Part model, mm, in its own coordinate system. Face numbers are marked on the shaded views. A direction names the side the tool comes from. Give positions to 0.01 mm unless a question says otherwise; leave off trailing zeros. Order: outer loops, then holes, each group sorted by start corner. A loop starts at its lowest first (then second) coordinate and runs counter-clockwise, first axis right, second up. Notation, with made-up numbers: (44.5, -28.75) - (89.5, -28.75) arc R18 cw to (89.5, -0.75) - close; hole circle Ø9 at (6.5, 0.5). An arc over 180 degrees is marked (long way). Use one line per item in the form item = value. Start each with the question number.
1. Tool access for the marked faces 1, 2 and 3: list every direction of +Z, -Z, +X, -X, +Y, -Y with a clear straight run to the whole face (end or side of a thin tool).
2. Band-saw the part on D-D, the plane x = 0. List the corners of the cut face in (y, z), plus the area to 3 significant figures.
3. Pull direction Z, two halves, no side cores. Call the marked faces 4, 5 and 6: +Z half, -Z half, draft (parallel to the pull), parting line (faces both ways), or undercut.
4. Pin check, flat tips, straight feed: P1, Ø4.5, axis at x = 0, z = -37.5, coming from the -Y side; P2, Ø2, axis at y = 2.5, z = 6.5, coming from the +X side; P3, Ø1.5, axis at x = -28.5, y = 1, coming from the +Z side. Stop position of each tip, or through.
5. Band-saw the part on C-C, the plane x = 7.5. List the corners of the cut face in (y, z).
6. Band-saw the part on B-B, the plane y = 1.3. List the corners of the cut face in (x, z), plus the area to 3 significant figures.
7. Drill centre lines: line 1 (Z direction, x = 1, y = 5.1); line 2 (X direction, y = 3.3, z = 14.5); line 3 (X direction, y = 5.25, z = 2.5). Where is each one in solid material? Low to high.
8. Band-saw the part on A-A, the plane z = 6. List the corners of the cut face in (x, y), plus the area to 3 significant figures.
from build123d import *

# Parameters (mm, degrees)
SKETCH1_R                = 17.5
BOSS_EXTRUDE1_DEPTH      = 5.5
SKETCH2_R                = 35
SKETCH2_R_2              = 17.5
SKETCH2_R_3              = 2.8
BOSS_EXTRUDE2_DEPTH      = 5.5
BOSS_EXTRUDE3_DEPTH      = 2
BOSS_EXTRUDE3_DEPTH_BACK = 5.5
SKETCH4_R                = 2.9
SKETCH5_R                = 5
BOSS_EXTRUDE4_DEPTH      = 1.5
SKETCH3_R                = 17.5
CUT_EXTRUDE1_DEPTH       = 10
SKETCH12_R               = 72.135852014
CUT_EXTRUDE2_DEPTH       = 22
FILLET1_R                = 10
SKETCH13_R               = 3.4
CUT_EXTRUDE3_DEPTH       = 10
SKETCH14_R               = 19
CUT_EXTRUDE4_DEPTH       = 10


with BuildPart() as part:
    # Sketch1 → Boss-Extrude1 (new body)
    with BuildSketch(Plane(origin=(0, 0, 0), x_dir=(1, 0, 0), z_dir=(0, 1, 0))):
        with Locations(Location((0, 0, 0), (0, 0, 270))):
            Circle(SKETCH1_R)
    extrude(amount=BOSS_EXTRUDE1_DEPTH)

    # Sketch2 → Boss-Extrude2 (add)
    with BuildSketch(Plane(origin=(0, 0, 0), x_dir=(1, 0, 0), z_dir=(0, 1, 0))):
        with Locations(Location((0, 0, 0), (0, 0, 270))):
            Circle(SKETCH2_R)
        Circle(SKETCH2_R_2, mode=Mode.SUBTRACT)
        with Locations(Location((0, 29, 0), (0, 0, 270))):
            Circle(SKETCH2_R_3, mode=Mode.SUBTRACT)
        with Locations(Location((25.11473671, -14.5, 0), (0, 0, 270))):
            Circle(SKETCH2_R_3, mode=Mode.SUBTRACT)
        with Locations(Location((-25.11473671, -14.5, 0), (0, 0, 270))):
            Circle(SKETCH2_R_3, mode=Mode.SUBTRACT)
    extrude(amount=BOSS_EXTRUDE2_DEPTH)

    # Sketch4 → Boss-Extrude3 (add, two sides: drawn at the far end of the back side and taken through both)
    with BuildSketch(Plane.XZ.offset(-BOSS_EXTRUDE3_DEPTH_BACK)):
        with Locations(Location((-25.11473671, 14.5, 0), (0, 0, 270))):
            Circle(SKETCH4_R)
        with Locations(Location((25.11473671, 14.5, 0), (0, 0, 270))):
            Circle(SKETCH4_R)
        with Locations(Location((0, -29, 0), (0, 0, 270))):
            Circle(SKETCH4_R)
    extrude(amount=BOSS_EXTRUDE3_DEPTH + BOSS_EXTRUDE3_DEPTH_BACK)

    # Sketch5 → Boss-Extrude4 (add)
    with BuildSketch(Plane(origin=(0, 5.5, 0), x_dir=(1, 0, 0), z_dir=(0, 1, 0))):
        with Locations((-30.453629482, -17.250404383)):
            Circle(SKETCH5_R)
        with Locations((0.28752632, 34.99881896)):
            Circle(SKETCH5_R)
        with Locations((30.166103162, -17.748414577)):
            Circle(SKETCH5_R)
    extrude(amount=-BOSS_EXTRUDE4_DEPTH)

    # Sketch3 → Cut-Extrude1 (cut)
    with BuildSketch(Plane(origin=(0, 5.5, 0), x_dir=(1, 0, 0), z_dir=(0, 1, 0))):
        with Locations(Location((0, 0, 0), (0, 0, 270))):
            Circle(SKETCH3_R)
    extrude(amount=-CUT_EXTRUDE1_DEPTH, mode=Mode.SUBTRACT)

    # Sketch12 → Cut-Extrude2 (cut)
    with BuildSketch(Plane(origin=(0, 5.5, 0), x_dir=(1, 0, 0), z_dir=(0, 1, 0))):
        Circle(SKETCH12_R)
        Polygon((0, 50), (-43.301270189, -25), (43.301270189, -25), align=None, mode=Mode.SUBTRACT)
    extrude(amount=-CUT_EXTRUDE2_DEPTH, mode=Mode.SUBTRACT)

    # Fillet1
    # the kernel refuses this fillet: 10 mm, written as the material it takes off along each edge
    with BuildSketch(Plane(origin=(-24.494897428, 18.7960859, 25), x_dir=(1, 0, 0), z_dir=(0, -1, 0))) as fillet1_piece_1_section:
        with BuildLine():
            CenterArc((4.494897428, -10), FILLET1_R, 90, 53.130102354)
            ThreePointArc((-3.505102572, -4), (-1.828638885, -1.933326291), (0, 0))
            Line((0, 0), (4.494897428, 0))
        make_face()
    fillet1_piece_1 = extrude(amount=32.0921718, mode=Mode.PRIVATE)
    fillet1_piece_1 = fillet1_piece_1 - Plane(origin=(-30.453629482, 4.75, 17.250404383), x_dir=(1, 0, 0), z_dir=(0, 1, 0)) * Cylinder(5, 83, mode=Mode.PRIVATE)
    add(fillet1_piece_1, mode=Mode.SUBTRACT)
    with BuildSketch(Plane(origin=(-24.494897428, 18.7960859, 25), x_dir=(1, 0, 0), z_dir=(0, -1, 0))) as fillet1_piece_2_section:
        with BuildLine():
            CenterArc((4.494897428, -10), FILLET1_R, 90, 53.130102354)
            ThreePointArc((-3.505102572, -4), (-1.828638885, -1.933326291), (0, 0))
            Line((0, 0), (4.494897428, 0))
        make_face()
    fillet1_piece_2 = extrude(amount=32.0921718, mode=Mode.PRIVATE)
    fillet1_piece_2 = split(fillet1_piece_2, bisect_by=Plane(origin=(-27.761621835, 4, 21.309124186), z_dir=(0, -1, 0)), keep=Keep.TOP, mode=Mode.PRIVATE)
    add(fillet1_piece_2, mode=Mode.SUBTRACT)
    with BuildSketch(Plane(origin=(24.494897428, 18.7960859, 25), x_dir=(-1, 0, 0), z_dir=(0, -1, 0))) as fillet1_piece_3_section:
        with BuildLine():
            CenterArc((4.494897428, 10), FILLET1_R, 216.869897646, 53.130102354)
            ThreePointArc((-3.505102572, 4), (-1.828638885, 1.933326291), (0, 0))
            Line((0, 0), (4.494897428, 0))
        make_face()
    fillet1_piece_3 = extrude(amount=32.0921718, mode=Mode.PRIVATE)
    fillet1_piece_3 = fillet1_piece_3 - Plane(origin=(30.166103162, 4.75, 17.748414577), x_dir=(1, 0, 0), z_dir=(0, 1, 0)) * Cylinder(5, 83, mode=Mode.PRIVATE)
    add(fillet1_piece_3, mode=Mode.SUBTRACT)
    with BuildSketch(Plane(origin=(24.494897428, 18.7960859, 25), x_dir=(-1, 0, 0), z_dir=(0, -1, 0))) as fillet1_piece_4_section:
        with BuildLine():
            CenterArc((4.494897428, 10), FILLET1_R, 216.869897646, 53.130102354)
            ThreePointArc((-3.505102572, 4), (-1.828638885, 1.933326291), (0, 0))
            Line((0, 0), (4.494897428, 0))
        make_face()
    fillet1_piece_4 = extrude(amount=32.0921718, mode=Mode.PRIVATE)
    fillet1_piece_4 = split(fillet1_piece_4, bisect_by=Plane(origin=(27.488157838, 4, 21.643747381), z_dir=(0, -1, 0)), keep=Keep.TOP, mode=Mode.PRIVATE)
    add(fillet1_piece_4, mode=Mode.SUBTRACT)
    with BuildSketch(Plane(origin=(-9.403186381, 18.7960859, -33.713203436), x_dir=(-0.5000000000000003, 0, 0.8660254037844386), z_dir=(0, -1, 0))) as fillet1_piece_5_section:
        with BuildLine():
            CenterArc((4.494897428, -10), FILLET1_R, 90, 53.130102354)
            ThreePointArc((-3.505102572, -4), (-1.828638885, -1.933326291), (0, 0))
            Line((0, 0), (4.494897428, 0))
        make_face()
    fillet1_piece_5 = extrude(amount=32.0921718, mode=Mode.PRIVATE)
    fillet1_piece_5 = fillet1_piece_5 - Plane(origin=(0.28752632, 4.75, -34.99881896), x_dir=(1, 0, 0), z_dir=(0, 1, 0)) * Cylinder(5, 83, mode=Mode.PRIVATE)
    add(fillet1_piece_5, mode=Mode.SUBTRACT)
    with BuildSketch(Plane(origin=(-9.403186381, 18.7960859, -33.713203436), x_dir=(-0.5000000000000003, 0, 0.8660254037844386), z_dir=(0, -1, 0))) as fillet1_piece_6_section:
        with BuildLine():
            CenterArc((4.494897428, -10), FILLET1_R, 90, 53.130102354)
            ThreePointArc((-3.505102572, -4), (-1.828638885, -1.933326291), (0, 0))
            Line((0, 0), (4.494897428, 0))
        make_face()
    fillet1_piece_6 = extrude(amount=32.0921718, mode=Mode.PRIVATE)
    fillet1_piece_6 = split(fillet1_piece_6, bisect_by=Plane(origin=(-4.57343196, 4, -34.696831852), z_dir=(0, -1, 0)), keep=Keep.TOP, mode=Mode.PRIVATE)
    add(fillet1_piece_6, mode=Mode.SUBTRACT)
    with BuildSketch(Plane(origin=(-33.898083809, 18.7960859, 8.713203436), x_dir=(0.32181469455231854, 0, 0.9468026734067654), z_dir=(0, -1, 0))) as fillet1_piece_7_section:
        with BuildLine():
            CenterArc((4.558658023, -9.971095222), FILLET1_R, 85.642603122, 53.130102354)
            Line((-2.962352352, -3.380617019), (0, 0))
            ThreePointArc((0, 0), (2.65921718, 0.101166725), (5.31843436, 0))
        make_face()
    fillet1_piece_7 = extrude(amount=32.0921718, mode=Mode.PRIVATE)
    fillet1_piece_7 = fillet1_piece_7 - Plane(origin=(-30.453629482, 4.75, 17.250404383), x_dir=(1, 0, 0), z_dir=(0, 1, 0)) * Cylinder(5, 86, mode=Mode.PRIVATE)
    add(fillet1_piece_7, mode=Mode.SUBTRACT)
    with BuildSketch(Plane(origin=(-33.898083809, 18.7960859, 8.713203436), x_dir=(0.32181469455231854, 0, 0.9468026734067654), z_dir=(0, -1, 0))) as fillet1_piece_8_section:
        with BuildLine():
            CenterArc((4.558658023, -9.971095222), FILLET1_R, 85.642603122, 53.130102354)
            Line((-2.962352352, -3.380617019), (0, 0))
            ThreePointArc((0, 0), (2.65921718, 0.101166725), (5.31843436, 0))
        make_face()
    fillet1_piece_8 = extrude(amount=32.0921718, mode=Mode.PRIVATE)
    fillet1_piece_8 = split(fillet1_piece_8, bisect_by=Plane(origin=(-32.488113984, 4, 12.9835693), z_dir=(0, -1, 0)), keep=Keep.TOP, mode=Mode.PRIVATE)
    add(fillet1_piece_8, mode=Mode.SUBTRACT)
    with BuildSketch(Plane(origin=(33.898083809, 18.7960859, 8.713203436), x_dir=(-0.5000000000000012, 0, -0.8660254037844382), z_dir=(0, -1, 0))) as fillet1_piece_9_section:
        with BuildLine():
            CenterArc((4.494897428, -10), FILLET1_R, 90, 53.130102354)
            ThreePointArc((-3.505102572, -4), (-1.828638885, -1.933326291), (0, 0))
            Line((0, 0), (4.494897428, 0))
        make_face()
    fillet1_piece_9 = extrude(amount=32.0921718, mode=Mode.PRIVATE)
    fillet1_piece_9 = fillet1_piece_9 - Plane(origin=(30.166103162, 4.75, 17.748414577), x_dir=(1, 0, 0), z_dir=(0, 1, 0)) * Cylinder(5, 83, mode=Mode.PRIVATE)
    add(fillet1_piece_9, mode=Mode.SUBTRACT)
    with BuildSketch(Plane(origin=(33.898083809, 18.7960859, 8.713203436), x_dir=(-0.5000000000000012, 0, -0.8660254037844382), z_dir=(0, -1, 0))) as fillet1_piece_10_section:
        with BuildLine():
            CenterArc((4.494897428, -10), FILLET1_R, 90, 53.130102354)
            ThreePointArc((-3.505102572, -4), (-1.828638885, -1.933326291), (0, 0))
            Line((0, 0), (4.494897428, 0))
        make_face()
    fillet1_piece_10 = extrude(amount=32.0921718, mode=Mode.PRIVATE)
    fillet1_piece_10 = split(fillet1_piece_10, bisect_by=Plane(origin=(32.335053795, 4, 13.387707666), z_dir=(0, -1, 0)), keep=Keep.TOP, mode=Mode.PRIVATE)
    add(fillet1_piece_10, mode=Mode.SUBTRACT)
    with BuildSketch(Plane(origin=(9.403186381, 18.7960859, -33.713203436), x_dir=(-0.9808625148174394, 0, -0.19470163590994477), z_dir=(0, -1, 0))) as fillet1_piece_11_section:
        with BuildLine():
            CenterArc((4.558658023, -9.971095222), FILLET1_R, 85.642603122, 53.130102354)
            Line((-2.962352352, -3.380617019), (0, 0))
            ThreePointArc((0, 0), (2.65921718, 0.101166725), (5.31843436, 0))
        make_face()
    fillet1_piece_11 = extrude(amount=32.0921718, mode=Mode.PRIVATE)
    fillet1_piece_11 = fillet1_piece_11 - Plane(origin=(0.28752632, 4.75, -34.99881896), x_dir=(1, 0, 0), z_dir=(0, 1, 0)) * Cylinder(5, 86, mode=Mode.PRIVATE)
    add(fillet1_piece_11, mode=Mode.SUBTRACT)
    with BuildSketch(Plane(origin=(9.403186381, 18.7960859, -33.713203436), x_dir=(-0.9808625148174394, 0, -0.19470163590994477), z_dir=(0, -1, 0))) as fillet1_piece_12_section:
        with BuildLine():
            CenterArc((4.558658023, -9.971095222), FILLET1_R, 85.642603122, 53.130102354)
            Line((-2.962352352, -3.380617019), (0, 0))
            ThreePointArc((0, 0), (2.65921718, 0.101166725), (5.31843436, 0))
        make_face()
    fillet1_piece_12 = extrude(amount=32.0921718, mode=Mode.PRIVATE)
    fillet1_piece_12 = split(fillet1_piece_12, bisect_by=Plane(origin=(4.999956146, 4, -34.627316681), z_dir=(0, -1, 0)), keep=Keep.TOP, mode=Mode.PRIVATE)
    add(fillet1_piece_12, mode=Mode.SUBTRACT)

    # Sketch13 → Cut-Extrude3 (cut)
    with BuildSketch(Plane(origin=(0, 5.5, 0), x_dir=(1, 0, 0), z_dir=(0, 1, 0))):
        with Locations(Location((0, 29, 0), (0, 0, 270))):
            Circle(SKETCH13_R)
        with Locations(Location((25.11473671, -14.5, 0), (0, 0, 270))):
            Circle(SKETCH13_R)
        with Locations(Location((-25.11473671, -14.5, 0), (0, 0, 270))):
            Circle(SKETCH13_R)
    extrude(amount=-CUT_EXTRUDE3_DEPTH, mode=Mode.SUBTRACT)

    # Sketch14 → Cut-Extrude4 (cut)
    with BuildSketch(Plane(origin=(0, 5.5, 0), x_dir=(1, 0, 0), z_dir=(0, 1, 0))):
        with Locations(Location((0, 0, 0), (0, 0, 270))):
            Circle(SKETCH14_R)
    extrude(amount=-CUT_EXTRUDE4_DEPTH, mode=Mode.SUBTRACT)


solid = part.part
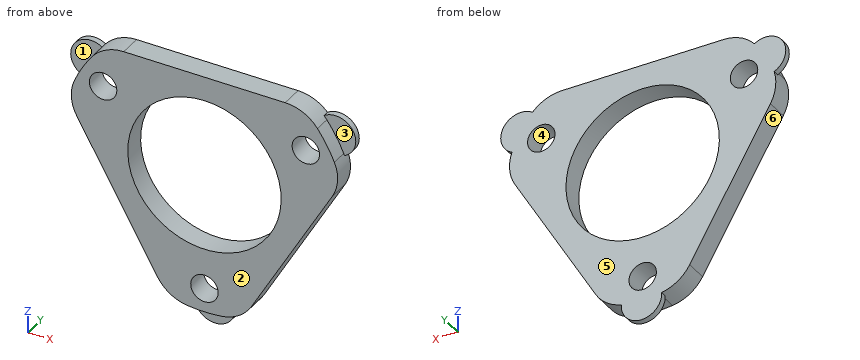
From the geometry:
q1.face_1 = +Z, -X, -Y
q1.face_2 = +Z, -Z, +X, -X, -Y
q1.face_3 = +Z, +X, -Y
q2.outline = (0, -35) - (4, -35) - (4, -39.99) - (5.5, -39.99) - (5.5, -32.4) - (0, -32.4) - close; (0, -25.6) - (5.5, -25.6) - (5.5, -19) - (0, -19) - close; (0, 19) - (5.5, 19) - (5.5, 25) - (0, 25) - close
q2.area = 91.1 mm²
q3.face_4 = undercut
q3.face_5 = draft
q3.face_6 = -Z half
q4.P1 = 4
q4.P2 = 32.72
q4.P3 = 21.32
q5.outline = (0, -33.75) - (5.5, -33.75) - (5.5, -17.46) - (0, -17.46) - close; (0, 17.46) - (5.5, 17.46) - (5.5, 25) - (0, 25) - close
q6.outline = (-32.19, 13.75) arc R10 ccw to (-31.65, 4.82) - (-11.65, -29.82) arc R10 ccw to (-4.19, -34.75) arc R35 ccw to (4.19, -34.75) arc R10 ccw to (11.65, -29.82) - (31.65, 4.82) arc R10 ccw to (32.19, 13.75) arc R35 ccw to (28, 21) arc R10 ccw to (20, 25) - (-20, 25) arc R10 ccw to (-28, 21) arc R35 ccw to start; hole circle Ø6.8 at (-25.11, 14.5); hole circle Ø38 at (0, 0); hole circle Ø6.8 at (0, -29); hole circle Ø6.8 at (25.11, 14.5)
q6.area = 1,580 mm²
q7.line_1 = -39.95 to -32.25, -25.75 to -18.97, 18.97 to 25
q7.line_2 = -31.86 to -28.51, -21.71 to -12.28, 12.28 to 21.71, 28.51 to 31.86
q7.line_3 = -30.31 to -18.83, 18.83 to 30.31
q8.outline = (-32.23, 0) - (-18.03, 0) - (-18.03, 5.5) - (-32.23, 5.5) - close; (18.03, 0) - (32.23, 0) - (32.23, 5.5) - (18.03, 5.5) - close
q8.area = 156 mm²
